```python
from build123d import *

# Parameters (mm, degrees)
SKETCH1_W           = 73
SKETCH1_H           = 80
SKETCH1_R           = 8.5
SKETCH1_R_2         = 4.5
SKETCH1_R_3         = 2.5
SKETCH1_W_2         = 28
SKETCH1_H_2         = 17
BOSS_EXTRUDE3_DEPTH = 2
SKETCH2_R           = 4
BOSS_EXTRUDE4_DEPTH = 2
SKETCH3_R           = 1.5
CUT_EXTRUDE1_DEPTH  = 10
SKETCH4_R           = 9.5
SKETCH4_R_2         = 8.5
BOSS_EXTRUDE5_DEPTH = 10
SKETCH5_R           = 5.360584101
SKETCH5_R_2         = 4.5
BOSS_EXTRUDE6_DEPTH = 5.2
SKETCH7_R           = 2.833966857
SKETCH7_R_2         = 2.5
BOSS_EXTRUDE7_DEPTH = 5.1


with BuildPart() as part:
    # Sketch1 → Boss-Extrude3 (new body)
    with BuildSketch(Plane.XY):
        with Locations((0, 10)):
            Rectangle(SKETCH1_W, SKETCH1_H)
        with Locations((-12.414904508, 21.373016215)):
            Circle(SKETCH1_R, mode=Mode.SUBTRACT)
        with Locations((14.085095492, 21.373016215)):
            Circle(SKETCH1_R, mode=Mode.SUBTRACT)
        with Locations((0.468085113, 38.834207529)):
            Circle(SKETCH1_R_2, mode=Mode.SUBTRACT)
        with Locations((-0.020060086, -19.374805823)):
            Circle(SKETCH1_R_3, mode=Mode.SUBTRACT)
        with Locations((0.468085113, -2.91182709)):
            Rectangle(SKETCH1_W_2, SKETCH1_H_2, mode=Mode.SUBTRACT)
    extrude(amount=BOSS_EXTRUDE3_DEPTH)

    # Sketch2 → Boss-Extrude4 (add)
    with BuildSketch(Plane.XY.offset(2)):
        with Locations((-36.5, 50)):
            Circle(SKETCH2_R)
        with Locations((36.5, 50)):
            Circle(SKETCH2_R)
        with Locations((36.5, -30)):
            Circle(SKETCH2_R)
        with Locations((-36.5, -30)):
            Circle(SKETCH2_R)
    extrude(amount=-BOSS_EXTRUDE4_DEPTH)

    # Sketch3 → Cut-Extrude1 (cut)
    with BuildSketch(Plane.XY.offset(2)):
        with Locations((-36.5, 50)):
            Circle(SKETCH3_R)
        with Locations((36.5, 50)):
            Circle(SKETCH3_R)
        with Locations((36.5, -30)):
            Circle(SKETCH3_R)
        with Locations((-36.5, -30)):
            Circle(SKETCH3_R)
    extrude(amount=-CUT_EXTRUDE1_DEPTH, mode=Mode.SUBTRACT)

    # Sketch4 → Boss-Extrude5 (add)
    with BuildSketch(Plane.XY.offset(2)):
        with Locations((-12.414904508, 21.373016215)):
            Circle(SKETCH4_R)
        with Locations((-12.414904508, 21.373016215)):
            Circle(SKETCH4_R_2, mode=Mode.SUBTRACT)
        with Locations((14.085095492, 21.373016215)):
            Circle(SKETCH4_R)
        with Locations((14.085095492, 21.373016215)):
            Circle(SKETCH4_R_2, mode=Mode.SUBTRACT)
    extrude(amount=BOSS_EXTRUDE5_DEPTH)

    # Sketch5 → Boss-Extrude6 (add)
    with BuildSketch(Plane(origin=(0, 0, 0), x_dir=(-1, 0, 0), z_dir=(0, 0, -1))):
        with Locations((-0.468085113, 38.834207529)):
            Circle(SKETCH5_R)
        with Locations((-0.468085113, 38.834207529)):
            Circle(SKETCH5_R_2, mode=Mode.SUBTRACT)
    extrude(amount=-BOSS_EXTRUDE6_DEPTH)

    # Sketch7 → Boss-Extrude7 (add)
    with BuildSketch(Plane.XY.offset(2)):
        with Locations((-0.020060086, -19.374805823)):
            Circle(SKETCH7_R)
        with Locations((-0.020060086, -19.374805823)):
            Circle(SKETCH7_R_2, mode=Mode.SUBTRACT)
    extrude(amount=BOSS_EXTRUDE7_DEPTH)


solid = part.part
```
Geometry: final body of the model. Coordinates: model frame, mm. A direction names the side the tool comes from. Coordinates: 2 decimals unless noted, no trailing zeros. Order: outer loops, then holes, each group sorted by start corner. A loop starts at its lowest first (then second) coordinate and runs counter-clockwise, first axis right, second up. Notation, with made-up numbers: (21.5, -30) -> (70.5, -30) arc R30 cw to (70.5, 2) -> close; hole circle Ø3 at (-35, 12.25). An arc over 180 degrees is marked (long way). Write each question's results on one line, items separated by ' | '. Start each with the question number.
1) First-contact query: pin 1 (1.7 mm diameter, centred on x = -0.5, y = -19, fed in from +Z); pin 2 (3 mm diameter, centred on x = 24.5, y = -19.5, fed in from +Z); pin 3 (0.6 mm diameter, centred on x = -7, z = 0.5, fed in from +Y); pin 4 (1 mm diameter, centred on y = 6.5, z = 1.5, fed in from +X). Flat tips, straight axial feed; report the tip coordinate or a pass-through.
2) Cut plane B-B, the plane x = 9.5. Output: boundary loops of the cut face in (y, z), and give its area (3 significant figures).
3) Mould query, pull axis Y, two halves, no side actions, for faces 6 (the cylindrical face through (-39.234, 52.92, 1.014)), 7 (the flat face through (0, -30, 1)), 8 (the flat face through (0, 50, 1)), 9 (the flat face through (-1, 11, 0)). Classes: released by +Y, released by -Y, zero draft, split by the parting line, or undercut.
4) Cut plane C-C, the plane y = 20. Output: boundary loops of the cut face in (x, z).
5) Set-up query: faces 1 (the flat face through (-1, 11, 2)), 2 (the flat face through (-21, 20, 12)), 3 (the cylindrical face through (39.42, 52.734, 1.014)), 4 (the flat face through (-36.5, 9, 1)), 5 (the flat face through (36.5, 9, 1)). Return all of +Z, -Z, +X, -X, +Y, -Y with unobstructed straight access to the full face (end or side cutting, diameter ignored); none if empty.
6) Cut plane A-A, the plane y = -8.5. Output: boundary loops of the cut face in (x, z).
7) Material intervals for line 1 along Y through (x, z) = (0, 3); line 2 along X through (y, z) = (15, 3.5); line 3 along Y through (x, z) = (-1, 5), sorted ascending.
Checks:
1) pin 1: through | pin 2: z = 2 | pin 3: y = 50 | pin 4: x = 36.5
2) outline: (-30, 0) -> (-11.41, 0) -> (-11.41, 2) -> (-30, 2) -> close; (5.59, 0) -> (14.22, 0) -> (14.22, 12) -> (13.05, 12) -> (13.05, 2) -> (5.59, 2) -> close; (28.53, 0) -> (50, 0) -> (50, 2) -> (29.69, 2) -> (29.69, 12) -> (28.53, 12) -> close | area: 121 mm^2
3) face 6: undercut | face 7: released by -Y | face 8: released by +Y | face 9: zero draft
4) outline: (-36.5, 0) -> (-20.8, 0) -> (-20.8, 12) -> (-21.82, 12) -> (-21.82, 2) -> (-36.5, 2) -> close; (-4.03, 0) -> (5.7, 0) -> (5.7, 12) -> (4.68, 12) -> (4.68, 2) -> (-3.01, 2) -> (-3.01, 12) -> (-4.03, 12) -> close; (22.47, 0) -> (36.5, 0) -> (36.5, 2) -> (23.49, 2) -> (23.49, 12) -> (22.47, 12) -> close
5) face 1: +Z | face 2: +Z, +X, -X, +Y, -Y | face 3: +Z, -Z | face 4: +Z, -Z, -X | face 5: +Z, -Z, +X
6) outline: (-36.5, 0) -> (-13.53, 0) -> (-13.53, 2) -> (-36.5, 2) -> close; (14.47, 0) -> (36.5, 0) -> (36.5, 2) -> (14.47, 2) -> close
7) line 1: -22.21 to -21.87, -16.87 to -16.54, 33.49 to 34.36, 43.31 to 44.17 | line 2: -19.46 to -18.04, -6.79 to -5.37, 7.04 to 8.46, 19.71 to 21.13 | line 3: -22.03 to -21.67, -17.07 to -16.72, 33.68 to 34.58, 43.09 to 43.99
